Autodesk Inventor part; units mm, degrees
ref_plane "Work Plane1" through (153.3626, 3.175, 315.1376) normal (0, 1, 0) x (1, 0, 0)
ref_plane "YZ Plane" through (0, 0, 0) normal (1, 0, 0) x (0, 1, 0)
ref_plane "XZ Plane" through (0, 0, 0) normal (0, 1, 0) x (-1, 0, 0)
ref_plane "Work Plane1" through (153.3626, 3.175, 315.1376) normal (0, 1, 0) x (1, 0, 0)
sketch "Sketch2" plane through (153.3626, 3.175, 315.1376) normal (0, 1, 0) x (1, 0, 0)
  line L0 (-69.85, 187.175) -> (-77.0435, 187.175)
  circle A0 centre (-88.9, 139.7) radius 2.65
  circle A1 centre (-88.9, 114.3) radius 2.65
  line L1 (-101.6, 142.5126) -> (-101.6, 66.6752)
  line L2 (-76.2, 34.5627) -> (-76.2, 28.5752)
  line L3 (-57.0148, 33.9239) -> (-71.3794, 33.9239) construction
  arc A2 (-82.55, 45.5613) -> (-79.375, 40.062) centre (-76.2, 45.5613) ccw
  line L4 (-76.2, 155.2126) -> (-76.2, 155.2126)
  line L5 (-19.05, 45.5613) -> (-19.05, 142.5127)
  line L6 (-25.4, 34.5627) -> (-25.4, 28.5752)
  arc A3 (-22.225, 40.062) -> (-25.4, 34.5627) centre (-19.05, 34.5627) ccw
  arc A4 (-22.225, 40.062) -> (-19.05, 45.5613) centre (-25.4, 45.5613) ccw
  arc A5 (19.0506, 161.5633) -> (0, 142.5127) centre (19.0506, 142.5127) ccw
  arc A6 (19.0506, 180.6133) -> (-19.05, 142.5127) centre (19.0506, 142.5127) ccw
  line L7 (-24.798, 231.625) -> (-24.798, 238.8185)
  circle A7 centre (22.0226, 250.7457) radius 2.65
  circle A8 centre (47.4226, 250.7457) radius 2.65
  arc A9 (133.2003, 174.2609) -> (132.8314, 250.6758) centre (133.2003, 212.4693) ccw
  line L8 (116.2139, 244.3252) -> (13.5144, 244.3252)
  arc A10 (133.2003, 186.9633) -> (133.2003, 237.9752) centre (133.2003, 212.4693) ccw
  line L9 (127.2124, 237.9752) -> (133.2003, 237.9752)
  arc A11 (121.7132, 241.1502) -> (127.2124, 237.9752) centre (127.2124, 244.3252) ccw
  arc A12 (121.7132, 241.1502) -> (116.2139, 244.3252) centre (116.2139, 237.9752) ccw
  line L10 (0.8144, 231.625) -> (-24.798, 231.625)
  line L11 (116.2145, 180.6133) -> (19.0506, 180.6133)
  arc A13 (127.213, 186.9633) -> (121.7138, 183.7883) centre (127.213, 180.6133) ccw
  arc A14 (116.2145, 180.6133) -> (121.7138, 183.7883) centre (116.2145, 186.9633) ccw
  line L12 (127.213, 186.9633) -> (133.2003, 186.9633)
  arc A15 (-24.798, 238.8185) -> (4.1198, 256.1306) centre (-34.9551, 288.5928) ccw
  arc A16 (18.7729, 263.0074) -> (4.1198, 256.1306) centre (18.7729, 243.9574) ccw
  line L13 (0, 142.5127) -> (0, 66.6752)
  arc A17 (-94.6727, 157.2075) -> (-101.6, 142.5126) centre (-82.55, 142.5126) ccw
  arc A18 (-94.6727, 157.2075) -> (-77.0435, 187.175) centre (-127, 196.3941) ccw
  line L14 (19.0506, 161.5633) -> (95.1006, 161.5633)
  line L15 (-101.6, 66.6752) -> (-101.6, 47.6252) construction
  line L16 (-101.6, 47.6252) -> (-88.9, 47.6252) construction
  line L17 (-88.9, 47.6252) -> (-88.9, 28.5752) construction
  spline S0 degree 3 poles (-101.6, 66.6752) (-101.6, 47.6252) (-88.9, 47.6252) (-88.9, 28.5752) knots 1 1 1 1 2 2 2 2
  spline S1 degree 3 poles (0, 66.6752) (0, 47.6252) (-12.7, 47.6252) (-12.7, 28.5752) knots 1 1 1 1 2 2 2 2
  line L18 (0, 66.6752) -> (0, 47.6252) construction
  line L19 (0, 47.6252) -> (-12.7, 47.6252) construction
  line L20 (-12.7, 47.6252) -> (-12.7, 28.5752) construction
  spline S2 degree 3 poles (94.6105, 263.0074) (113.6596, 263.1913) (113.7823, 250.4919) (132.8314, 250.6758) knots 1 1 1 1 2 2 2 2
  line L21 (94.6105, 263.0074) -> (113.6596, 263.1913) construction
  line L22 (113.6596, 263.1913) -> (113.7823, 250.4919) construction
  line L23 (113.7823, 250.4919) -> (132.8314, 250.6758) construction
  spline S3 degree 3 poles (95.1006, 161.5633) (114.1506, 161.5633) (114.1506, 174.2609) (133.2003, 174.2609) knots 1 1 1 1 2 2 2 2
  line L24 (95.1006, 161.5633) -> (114.1506, 161.5633) construction
  line L25 (114.1506, 161.5633) -> (114.1506, 174.2609) construction
  line L26 (114.1506, 174.2609) -> (133.2003, 174.2609) construction
  circle A19 centre (-88.9, 88.9) radius 2.65
  circle A20 centre (-88.9, 63.5) radius 2.65
  circle A21 centre (-82.55, 28.5752) radius 2.65
  circle A22 centre (-19.05, 28.5752) radius 2.65
  circle A23 centre (-12.7, 63.5) radius 2.65
  circle A24 centre (-12.7, 88.9) radius 2.65
  circle A25 centre (-12.7, 114.3) radius 2.65
  circle A26 centre (-12.7, 139.7) radius 2.65
  circle A27 centre (22.075, 174.475) radius 2.65
  circle A28 centre (47.475, 174.475) radius 2.65
  circle A29 centre (72.875, 174.475) radius 2.65
  circle A30 centre (98.275, 174.475) radius 2.65
  circle A31 centre (133.2, 180.825) radius 2.65
  circle A32 centre (133.2, 244.325) radius 2.65
  circle A33 centre (98.2226, 250.7457) radius 2.65
  circle A34 centre (72.8226, 250.7457) radius 2.65
  arc A35 (-88.9, 28.5752) -> (-12.7, 28.5752) centre (-50.8, 28.5752) ccw
  line L27 (94.6105, 263.0074) -> (18.7729, 263.0074)
  line L28 (-69.85, 187.175) -> (-69.85, 161.5626)
  line L29 (-82.55, 148.8626) -> (-82.55, 45.5613)
  arc A36 (-76.2, 34.5627) -> (-79.375, 40.062) centre (-82.55, 34.5627) ccw
  arc A37 (0.8144, 231.625) -> (7.1644, 237.9751) centre (0.8144, 237.975) ccw
  arc A38 (13.5144, 244.3252) -> (7.1644, 237.9751) centre (13.5144, 237.9752) ccw
  arc A39 (-76.2, 155.2126) -> (-69.85, 161.5626) centre (-76.2, 161.5626) ccw
  arc A40 (-76.2, 155.2126) -> (-82.55, 148.8626) centre (-76.2, 148.8626) ccw
  arc A41 (-76.2, 28.5752) -> (-25.4, 28.5752) centre (-50.8, 28.5752) ccw
  point P0 (19.2624, 180.825)
  point P1 (-19.05, 142.5126)
  point P2 (-153.3626, 315.1376)
  dimension "d62" = 5.3
  dimension "d64" = 7.1935
  dimension "d65" = 25.6124
  dimension "d72" = 12.7
  dimension "d73" = 19.05
  dimension "d74" = 19.05
  dimension "d75" = 6.4205
  dimension "d76" = 25.4
  dimension "d77" = 25.4
  dimension "d78" = 25.4
  dimension "d104" = 6.35
  dimension "d105" = 6.35
  dimension "d106" = 6.35
  dimension "d107" = 6.35
  dimension "d109" = 6.35
  dimension "d110" = 6.35
  dimension "d111" = 19.05
  dimension "d112" = 19.05
  dimension "d114" = 34.9248
  dimension "d115" = 31.75
  dimension "d116" = 25.4
  dimension "d117" = 25.4
  dimension "d118" = 25.4
  dimension "d122" = 38.1
  dimension "d124" = 5.3
  dimension "d125" = 6.35
  dimension "d126" = 6.35
  dimension "d127" = 6.35
  dimension "d128" = 5.9875
  dimension "d129" = 12.7
  dimension "d130" = 19.05
  dimension "d131" = 19.05
  dimension "d132" = 16.9861
  dimension "d133" = 6.35
  dimension "d134" = 96.9515
  dimension "d135" = 5.4993
  dimension "d136" = 25.4
  dimension "d137" = 102.5626
  dimension "d138" = 286.5624
  dimension "d139" = 25.4
  dimension "d140" = 5.9875
  dimension "d141" = 12.7
  dimension "d142" = 12.7
  dimension "d143" = 19.05
  dimension "d144" = 19.05
  dimension "d145" = 12.7
  dimension "d146" = 25.4
  dimension "d147" = 19.0506
  dimension "d148" = 25.4
  dimension "d149" = 25.4
  dimension "d150" = 25.4
  dimension "d151" = 5.3
  dimension "d152" = 19.05
  dimension "d153" = 12.6976
  dimension "d154" = 19.0497
  dimension "d155" = 38.2083
  dimension "d156" = 25.5059
  dimension "d157" = 6.35
  dimension "d158" = 6.35
  dimension "d159" = 97.1639
  dimension "d160" = 10.9985
  dimension "d161" = 5.4993
  dimension "d162" = 5.9873
  dimension "d163" = 5.3
extrude "Extrusion2" add sketch "Sketch2" along normal blind 34.417
properties part number "Gearbox Cover Large"
The model under review builds one solid part; all positions refer to its coordinate system, in mm. A direction names the side the tool comes from. Round coordinates to 2 decimals unless told otherwise and drop trailing zeros. Order: outer loops, then holes, each group sorted by start corner. A loop starts at its lowest first (then second) coordinate and runs counter-clockwise, first axis right, second up. Notation, with made-up numbers: (33, 7) -> (77, 7) arc R17 ccw to (77, 40) -> close; hole circle Ø2 at (29.25, -17.75). An arc over 180 degrees is marked (long way). Return JSON: item names as keys, results as strings.
1. For L1, parallel to Z at x = 220.5, y = 25.5; L2, parallel to X at y = 28, z = 216; L3, parallel to Z at x = 310, y = 35, list the stretches that pass through material, from the lowest coordinate up. Write a range as [from, to].
Answer block:
{"L1": "z = [52.13, 70.81], [134.52, 153.57]", "L2": "x = [51.76, 70.81], [134.31, 153.36]", "L3": "z = [72.49, 92.61], [112.73, 132.84]"}
2. Take a section at D-D (x = 93). Write out the cut boundary in (y, z) (3 decimals), then the cut area to 3 significant figures.
Answer block:
{"outline": "(3.175, 310.094) -> (37.592, 310.094) -> (37.592, 323.443) -> (3.175, 323.443) -> close", "area": "459 mm²"}
3. Insertion check: P1, Ø7.5, axis at x = 135, y = 14, coming from the +Z side; P2, Ø2, axis at y = 24, z = 115, coming from the +X side; P3, Ø6, axis at x = 140.66, z = 226.24, coming from the +Y side; P4, Ø6.5, axis at y = 19.5, z = 283.5, coming from the +X side. Each pin has a flat end and moves straight along its axis. Give the tip position at first contact, or say it passes through.
Answer block:
{"P1": "stops at z = 311.64", "P2": "stops at x = 323.05", "P3": "stops at y = 37.59", "P4": "stops at x = 141.21"}
4. Take a section at C-C (y = 11.5). State how many separate pieces and enclosed holes the cut face has, then the cut area to 3 significant figures.
Answer block:
{"separate pieces": "1", "enclosed holes": "20", "area": "12,300 mm²"}
5. Take a section at A-A (z = 213). Write out the cut boundary in (x, y) (3 decimals), then the cut area to 3 significant figures.
Answer block:
{"outline": "(51.763, 3.175) -> (70.813, 3.175) -> (70.813, 37.592) -> (51.763, 37.592) -> close; (134.313, 3.175) -> (153.363, 3.175) -> (153.363, 37.592) -> (134.313, 37.592) -> close", "area": "1,310 mm²"}
6. The part is to be moulded in two halves that separate along X. For faces 5 (the face through (157, 3.175, 157)), 6 (the face through (312.063, 20.143, 102.107)), 7 (the face through (158.8, 20.1, 159.3)), say which applies: +X half, -X half, draft (parallel to the pull), parting line (faces both ways), or undercut.
Answer block:
{"face 5": "draft", "face 6": "undercut", "face 7": "+X half"}
7. Take a section at B-B (x = 181.5). Write out the cut boundary in (y, z) (3 decimals), then the cut area to 3 significant figures.
Answer block:
{"outline": "(3.175, 52.13) -> (37.592, 52.13) -> (37.592, 70.812) -> (3.175, 70.812) -> close; (3.175, 134.524) -> (37.592, 134.524) -> (37.592, 153.574) -> (3.175, 153.574) -> close", "area": "1,300 mm²"}
8. For faces 1 (the face through (128.565, 20, 80)), 2 (the face through (222, 20, 134.524)), 3 (the face through (127.963, 20, 284)), 4 (the face through (210, 20, 153.574)), list the 3-axis set-ups (+Z, -Z, +X, -X, +Y, -Y) from which the entire face can be reached by the end or side of a thin tool; tool diameter is ignored.
Answer block:
{"face 1": "-Z, -X, +Y, -Y", "face 2": "+Y, -Y", "face 3": "-Z, +Y, -Y", "face 4": "+Z, +X, +Y, -Y"}
